Source: CAD feature listing. Evaluate the final solid. Frame: model axes, mm. A direction names the side the tool comes from. Round coordinates to 2 decimals unless told otherwise and drop trailing zeros. Loops run counter-clockwise (first coordinate to the right, second up) from the corner with the lowest first, then second, coordinate; pieces in that order, holes last.
Item 1: Access query for faces 1 (the cylindrical face through (-23.977, -1.055, 1.986)), 2 (the cylindrical face through (24.141, -23.942, 1.479)), 3 (the flat face through (-14, 20, 0)). Directions: +Z, -Z, +X, -X, +Y, -Y. A direction counts if a zero-diameter tool reaches every point of the face in a straight line with its end or side. Return the directions, or none.
Item 2: Section query C-C on z = -5.5. Return loops of the section in (x, y), then the cut area to 3 significant figures.
Item 3: Ray query, L1, parallel to Y at x = 0, z = 2.55; L2, parallel to Z at x = -18.5, y = 1; L3, parallel to Z at x = -24.5, y = -17. Return the intervals inside material, ascending.
Item 4: First-contact query: P1, Ø1.5, axis at x = 9, z = -2, coming from the +Y side; P2, Ø5, axis at x = -0.5, z = -4.5, coming from the +Y side; P3, Ø2, axis at x = 10.5, z = -16.5, coming from the +Y side. Flat tips, straight axial feed; report the tip coordinate or a pass-through.
Item 5: Section query A-A on x = 0. Return loops of the section in (y, z), then the cut area to 3 significant figures.
Item 6: Pull-direction query (Y, two-part tool) for faces 4 (the flat face through (0, 30, 1)), 5 (the cylindrical face through (-19.32, 21.75, 1.48)), 6 (the flat face through (0, -30, 1)); classes: released by +Y, released by -Y, zero draft, split by the parting line, or undercut.
Item 7: Section query D-D on x = -20. Return loops of the section in (y, z).
Autodesk Inventor part; units mm, degrees
ref_plane "YZ Plane" through (0, 0, 0) normal (1, 0, 0) x (0, 1, 0)
ref_plane "XZ Plane" through (0, 0, 0) normal (0, 1, 0) x (-1, 0, 0)
ref_plane "XY Plane" through (0, 0, 0) normal (0, 0, 1) x (1, 0, 0)
sketch "Sketch1" plane through (0, 0, 0) normal (0, 0, 1) x (1, 0, 0)
  circle A0 centre (0, 0) radius 23.5 construction
  circle A1 centre (0, 0) radius 34 construction
  line L0 (30, 30) -> (-30, 30) construction
  line L1 (-30, 30) -> (-30, -30) construction
  line L2 (-30, -30) -> (30, -30) construction
  line L3 (30, -30) -> (30, 30) construction
  line L4 (30, 30) -> (-30, -30) construction
  line L5 (-30, 30) -> (30, -30) construction
  circle A2 centre (20.1525, 20.1525) radius 4 construction
  circle A3 centre (20.1525, 20.1525) radius 1.8
  arc A4 (30, 16) -> (16, 30) centre (0, 0) ccw
  line L6 (30, 16) -> (30, -16)
  circle A5 centre (0, 0) radius 24
  arc A6 (-16, 30) -> (-30, 16) centre (0, 0) ccw
  line L7 (-16, 30) -> (16, 30)
  circle A7 centre (-20.1525, 20.1525) radius 1.8
  arc A8 (-30, -16) -> (-16, -30) centre (0, 0) ccw
  line L8 (-30, -16) -> (-30, 16)
  circle A9 centre (-20.1525, -20.1525) radius 1.8
  arc A10 (16, -30) -> (30, -16) centre (0, 0) ccw
  line L9 (16, -30) -> (-16, -30)
  circle A11 centre (20.1525, -20.1525) radius 1.8
  line L10 (-35, 35) -> (35, 35)
  line L11 (35, 35) -> (35, -35)
  line L12 (35, -35) -> (-35, -35)
  line L13 (-35, -35) -> (-35, 35)
  line L14 (-35, 35) -> (35, -35) construction
  line L15 (35, 35) -> (-35, -35) construction
  point P0 (-16, -30)
  point P1 (30, -16)
  point P2 (16, 30)
  dimension "d2" = 60
  dimension "d3" = 60
  dimension "d4" = 68
  dimension "d5" = 47
  dimension "d6" = 8
  dimension "d7" = 28.5
  dimension "d8" = 3.6
  dimension "d9" = 48
  dimension "d10" = 360
  dimension "d11" = 70
  dimension "d12" = 70
extrude "Extrusion1" add sketch "Sketch1" along normal blind 3 contours L6 A10 L9 A8 L8 A6 L7 A4
extrude "Extrusion2" add sketch "Sketch1" along normal blind 1 contours A5
extrude "Extrusion3" add sketch "Sketch1" against normal blind 22 contours A5
properties part number "tweetwe"
Data:
1. face 1: +Z
1. face 2: +Z, -Z, +X, -Y
1. face 3: -Z
2. outline: circle Ø48 at (0, 0)
2. area: 1,810 mm2
3. L1: y = -30 to -24, 24 to 30
3. L2: z = -22 to 1
3. L3: z = 0 to 3
4. P1: stops at y = 22.54
4. P2: stops at y = 24
4. P3: stops at y = 22.04
5. outline: (-30, 0) - (-24, 0) - (-24, -22) - (24, -22) - (24, 0) - (30, 0) - (30, 3) - (24, 3) - (24, 1) - (-24, 1) - (-24, 3) - (-30, 3) - close
5. area: 1,140 mm2
6. face 4: released by +Y
6. face 5: undercut
6. face 6: released by -Y
7. outline: (-27.5, 0) - (-21.95, 0) - (-21.95, 3) - (-27.5, 3) - close; (-18.36, 0) - (-13.27, 0) - (-13.27, -22) - (13.27, -22) - (13.27, 0) - (18.36, 0) - (18.36, 3) - (13.27, 3) - (13.27, 1) - (-13.27, 1) - (-13.27, 3) - (-18.36, 3) - close; (21.95, 0) - (27.5, 0) - (27.5, 3) - (21.95, 3) - close
